For this review, take the finished solid that the model builds, in its own axes (mm). A direction names the side the tool comes from. Coordinates: 2 decimals unless noted, no trailing zeros. Loops run counter-clockwise (first coordinate to the right, second up) from the corner with the lowest first, then second, coordinate; pieces in that order, holes last. Notation, with made-up numbers: M -18,71 L 19,71 A12 cw 19,81 Z; hole C -22,23.25 d10. An arc over 180 degrees is marked long. Answer as a JSON object with one key per item and string values. Group by question number.
Item 1: Insertion check: pin 1 (14.5 mm diameter, centred on y = 14, z = 10, fed in from +X); pin 2 (9 mm diameter, centred on y = 14, z = -6, fed in from -X); pin 3 (3 mm diameter, centred on x = 35.5, y = 19.5, fed in from -Z); pin 4 (7.5 mm diameter, centred on x = -11, y = 7, fed in from +Z). Each pin has a flat end and moves straight along its axis. Give the tip position at first contact, or say it passes through.
Item 2: Add section D-D (x = -9). State the section outline as (y, z) points, then the cut area to 3 significant figures.
Item 3: Add section A-A (y = 2.75). State the section outline as (x, z) points, then the cut area to 3 significant figures.
Item 4: Tool access review of faces 4 (the face through (0.483, 16.173, 8.541)), 5 (the face through (-36.43, 12.65, 18.96)), 6 (the face through (37, 13, -5)), 7 (the face through (36.43, 12.65, 18.87)), 8 (the face through (-1, 4.25, -35)): name each direction out of +Z, -Z, +X, -X, +Y, -Y from which nothing blocks a thin tool from reaching the whole face with its end or side.
Item 5: Add section C-C (z = -12.5). State the section outline as (x, y) points, then the cut area to 3 significant figures.
Item 6: Add section B-B (x = 40). State the section outline as (y, z) points, then the cut area to 3 significant figures.
Item 7: Wall thickness on L1, parallel to X at y = 10, z = -13.5; L2, parallel to Z at x = -2, y = 2; L3, parallel to Y at x = -8, z = 2.5: over which ranges is each line inside the solid? List them lowest first. Write a range as from..to.
Item 8: Mouldability with a two-part tool opening along Z and no side actions: class faces 1 (the face through (-1, 0, 27)), 2 (the face through (-45, 2.15, 38.07)), 3 (the face through (-38.66, 2.1, -29.89)) as +Z half, -Z half, draft (parallel to the pull), parting line (faces both ways), or undercut.
from build123d import *

# Parameters (mm, degrees)
F0_W     = 93
F0_H     = 79
F0_R     = 2.5
F0_W_2   = 69
F0_H_2   = 49
F1_DEPTH = 4.25
F2_W     = 74
F2_H     = 54
F2_W_2   = 69
F2_H_2   = 49
F3_DEPTH = 20
F6_DEPTH = 83.501
F8_DEPTH = 71.5
F9_R     = 5
F10_R    = 2


with BuildPart() as f1:
    # F0 (on Front) → F1 (new body)
    with BuildSketch(Plane.XZ):
        Rectangle(F0_W, F0_H)
        with Locations((-40, -32)):
            Circle(F0_R, mode=Mode.SUBTRACT)
        with Locations((40, -32)):
            Circle(F0_R, mode=Mode.SUBTRACT)
        with Locations((-40, 32)):
            Circle(F0_R, mode=Mode.SUBTRACT)
        Rectangle(F0_W_2, F0_H_2, mode=Mode.SUBTRACT)
        with Locations((40, 32)):
            Circle(F0_R, mode=Mode.SUBTRACT)
    extrude(amount=-F1_DEPTH)

    # F2 (on face) → F3 (join)
    with BuildSketch(Plane(origin=(0, 4.25, 0), x_dir=(-1, 0, 0), z_dir=(0, 1, 0))):
        Rectangle(F2_W, F2_H)
        Rectangle(F2_W_2, F2_H_2, mode=Mode.SUBTRACT)
    extrude(amount=F3_DEPTH)

    # F5 (on face) → F6 (cut, through all)
    with BuildSketch(Plane.YZ.offset(37)):
        Polygon((24.25, 29.4060515452), (13.25, 29.4060515452), (13.25, 15), (24.25, 4), align=None)
    extrude(amount=-F6_DEPTH, mode=Mode.SUBTRACT)

    # F7 (on face) → F8 (join, through all)
    with BuildSketch(Plane.YZ.offset(37)):
        Polygon((13.25, 27), (10.75, 27), (10.75, 13.9644660941), (21.75, 2.9644660941), (21.75, -27), (24.25, -27), (24.25, 4), (13.25, 15), align=None)
    extrude(amount=-F8_DEPTH)

    # F9
    f9_edges = [f1.edges().sort_by_distance(p)[0] for p in [
        (37, 14.25, -27),
        (37, 8.75, 27),
        (-37, 8.75, 27),
        (-37, 14.25, -27),
        (-46.5, 2.125, 39.5),
        (-46.5, 2.125, -39.5),
        (46.5, 2.125, 39.5),
        (46.5, 2.125, -39.5),
        (-34.5, 5.375, 24.5),
        (34.5, 5.375, 24.5),
        (34.5, 10.875, -24.5),
        (-34.5, 10.875, -24.5),
    ]]
    fillet(f9_edges, radius=F9_R)

    # F10
    f10_edges = [f1.edges().sort_by_distance(p)[0] for p in [
        (37, 13.25, 18.5),
        (37, 18.75, 9.5),
        (37, 24.25, -9),
        (-37, 18.75, 9.5),
        (0, 13.25, 27),
        (0, 24.25, -27),
        (-37, 24.25, -9),
        (-37, 13.25, 18.5),
        (0, 24.25, 4),
        (0, 13.25, 15),
    ]]
    fillet(f10_edges, radius=F10_R)


solid = f1.part
From the geometry:
{
 "1": {"pin 1": "stops at x = 37", "pin 2": "stops at x = -37", "pin 3": "stops at z = -26.58", "pin 4": "stops at z = 39.5"},
 "2": {"outline": "M 0,-39.5 L 4.25,-39.5 L 4.25,-27 L 22.25,-27 A2 ccw 24.25,-25 L 24.25,3.17 A2 ccw 23.66,4.59 L 13.84,14.41 A2 cw 13.25,15.83 L 13.25,25 A2 ccw 11.25,27 L 4.25,27 L 4.25,39.5 L 0,39.5 L 0,24.5 L 10.75,24.5 L 10.75,13.96 L 21.75,2.96 L 21.75,-24.5 L 0,-24.5 Z", "area": "332 mm²"},
 "3": {"outline": "M -46.5,-34.5 A5 ccw -41.5,-39.5 L 41.5,-39.5 A5 ccw 46.5,-34.5 L 46.5,34.5 A5 ccw 41.5,39.5 L -41.5,39.5 A5 ccw -46.5,34.5 Z; hole C -40,-32 d5; hole C -40,32 d5; hole M -34.5,-19.5 A5 ccw -29.5,-24.5 L 29.5,-24.5 A5 ccw 34.5,-19.5 L 34.5,19.5 A5 ccw 29.5,24.5 L -29.5,24.5 A5 ccw -34.5,19.5 Z; hole C 40,-32 d5; hole C 40,32 d5", "area": "3,890 mm²"},
 "4": {"face 4": "-Y", "face 5": "+Z, -X, +Y", "face 6": "+Z, -Z, +X, +Y", "face 7": "+Z, +X, +Y", "face 8": "+Y"},
 "5": {"outline": "M -46.5,0 L -34.5,0 L -34.5,21.75 L 34.5,21.75 L 34.5,0 L 46.5,0 L 46.5,4.25 L 37,4.25 L 37,22.25 A2 ccw 35,24.25 L -35,24.25 A2 ccw -37,22.25 L -37,4.25 L -46.5,4.25 Z", "area": "373 mm²"},
 "6": {"outline": "M 0,-39.5 L 4.25,-39.5 L 4.25,-34.5 L 0,-34.5 Z; M 0,-29.5 L 4.25,-29.5 L 4.25,29.5 L 0,29.5 Z; M 0,34.5 L 4.25,34.5 L 4.25,39.5 L 0,39.5 Z", "area": "293 mm²"},
 "7": {"L1": "x = -37..-34.5, 34.5..37", "L2": "z = -39.5..-24.5, 24.5..39.5", "L3": "y = 21.75..24.25"},
 "8": {"face 1": "draft", "face 2": "+Z half", "face 3": "undercut"}
}
